Build history of the part. All positions in model axes, mm. Give positions to 0.01 mm unless a question says otherwise; leave off trailing zeros. One line per item, written item: value. Start each with the question number.
from build123d import *

# Parameters (mm, degrees)
SKETCH1_W                = 1508
SKETCH1_H                = 40
BOSS_EXTRUDE1_DEPTH      = 1.5
BOSS_EXTRUDE1_DEPTH_BACK = 1.5
FILLET1_R                = 0.35
SKETCH2_W                = 4
SKETCH2_H                = 20
CUT_EXTRUDE1_DEPTH       = 4


with BuildPart() as part:
    # Sketch1 → Boss-Extrude1 (new body, two sides)
    with BuildSketch(Plane(origin=(0, 0, 0), x_dir=(1, 0, 0), z_dir=(0, 1, 0))) as boss_extrude1_sk:
        Rectangle(SKETCH1_W, SKETCH1_H)
    extrude(amount=BOSS_EXTRUDE1_DEPTH)
    extrude(boss_extrude1_sk.sketch, amount=-BOSS_EXTRUDE1_DEPTH_BACK)

    # Fillet1
    fillet1_edges = [part.edges().sort_by_distance(p)[0] for p in [
        (0, 1.5, -20),
        (0, 1.5, 20),
        (0, -1.5, 20),
        (0, -1.5, -20),
    ]]
    fillet(fillet1_edges, radius=FILLET1_R)

    # Sketch2 → Cut-Extrude1 (cut, through all)
    with BuildSketch(Plane(origin=(0, 1.5, 0), x_dir=(1, 0, 0), z_dir=(0, 1, 0))):
        with Locations((530.92, 10)):
            Rectangle(SKETCH2_W, SKETCH2_H)
        with Locations((706.83, 10)):
            Rectangle(SKETCH2_W, SKETCH2_H)
        with Locations((355.01, 10)):
            Rectangle(SKETCH2_W, SKETCH2_H)
        with Locations((179.1, 10)):
            Rectangle(SKETCH2_W, SKETCH2_H)
        with Locations((3.19, 10)):
            Rectangle(SKETCH2_W, SKETCH2_H)
        with Locations((-172.72, 10)):
            Rectangle(SKETCH2_W, SKETCH2_H)
        with Locations((-348.63, 10)):
            Rectangle(SKETCH2_W, SKETCH2_H)
        with Locations((-524.54, 10)):
            Rectangle(SKETCH2_W, SKETCH2_H)
        with Locations((-700.45, 10)):
            Rectangle(SKETCH2_W, SKETCH2_H)
    extrude(amount=-CUT_EXTRUDE1_DEPTH, mode=Mode.SUBTRACT)


solid = part.part
1) Probe line 1 along Z through (x, y) = (617.5, -1.3). List the from-to ranges inside material, lowest first. Write a range as from..to.
2) Drop a flat-ended pin along its axis: P1, Ø1.5, axis at x = -348, y = -0.5, coming from the -Z side. Give the stop position or say it passes through.
3) Band-saw the part on A-A (z = -11). Count the separate pieces of the cut face and the enclosed holes in it, then the cut area to 3 significant figures.
Model answer:
1. line 1: z = -19.97..19.97
2. P1: stops at z = 0
3. separate pieces: 10
3. enclosed holes: 0
3. area: 4,420 mm²
